Could you check a few things on this model? Use its own coordinates, in mm. Face numbers are marked on the shaded views. A direction names the side the tool comes from. Coordinates: 2 decimals unless noted, no trailing zeros. Loops run counter-clockwise (first coordinate to the right, second up) from the corner with the lowest first, then second, coordinate; pieces in that order, holes last.
1) Will these pins go through, and if not, where does the flat tip stop? P1, Ø6.5, axis at x = 0.5, z = 1, coming from the -Y side; P2, Ø6, axis at y = 11.5, z = -0.5, coming from the +X side; P3, Ø2, axis at x = 5, y = 18, coming from the -Z side; P4, Ø1.5, axis at y = 40, z = 3, coming from the +X side.
2) If I drill on line 1 along X through (y, z) = (1.45, 0); line 2 along Y through (x, z) = (0.25, 3.25); line 3 along Y through (x, z) = (-6.75, -1.75), over which ranges is the centre line in solid material (lowest first)?
3) Imagine slicing it at B-B on x = -6.5. Give the number of separate pieces and of enclosed holes in the cut face, plus the area to 3 significant figures.
4) For the marked faces 1 and 2, which set-ups out of +Z, -Z, +X, -X, +Y, -Y let a thin tool reach every point of the face, with its end or its side?
5) Imagine slicing it at A-A on y = 18. Please give me the cut outline in (x, z), plus the area to 3 significant figures.
```python
from build123d import *


with BuildPart() as f1:
    # F0 (on Right) → F1 (revolve)
    with BuildSketch(Plane.YZ):
        Polygon((28.85, 6), (0, 6), (0, 2.25), (1.75, 2.25), (1.75, 4), (2.75, 4), (2.75, 2.25), (37.75, 2.25), (39.049038, 0), (49, 0), (50, 0.57735), (50, 8), (49, 9), (48.5, 9), (48.5, 6), (46.95, 6), (46.95, 9), (45.95, 9), (45.95, 6), (44.4, 6), (44.4, 9), (43.4, 9), (43.4, 6), (41.85, 6), (41.85, 9), (31.85, 9), align=None)
    revolve(axis=Axis((0, 25.938479, 0), (0, 1, 0)))


solid = f1.part
```
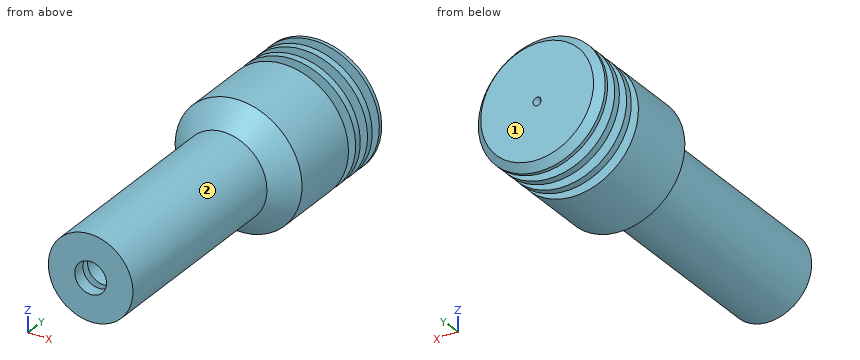
Filled in:
1. P1: stops at y = 0
1. P2: stops at x = 6
1. P3: stops at z = -4.47
1. P4: stops at x = 8.71
2. line 1: x = -6 to -2.25, 2.25 to 6
2. line 2: y = 0 to 1.75, 2.75 to 50
2. line 3: y = 29.82 to 41.85, 43.4 to 44.4, 45.95 to 46.95, 48.5 to 50
3. separate pieces: 4
3. enclosed holes: 0
3. area: 187 mm2
4. face 1: +Z, -Z, +X, -X, +Y
4. face 2: -Y
5. outline: circle Ø12 at (0, 0); hole circle Ø4.5 at (0, 0)
5. area: 97.2 mm2
